Answer from the drawing. Dimensions are ordinates in mm from the lowest x, y and z of the part. A direction names the side the tool comes from. Give positions to 0.01 mm unless a question says otherwise; leave off trailing zeros. Order: outer loops, then holes, each group sorted by start corner. A loop starts at its lowest first (then second) coordinate and runs counter-clockwise, first axis right, second up. Notation, with made-up numbers: M 18,76.25 L 32,76.25 A4 cw 32,80.25 Z; hole C 69.25,20.5 d4. An arc over 180 degrees is marked long. One line per item, written item: value.
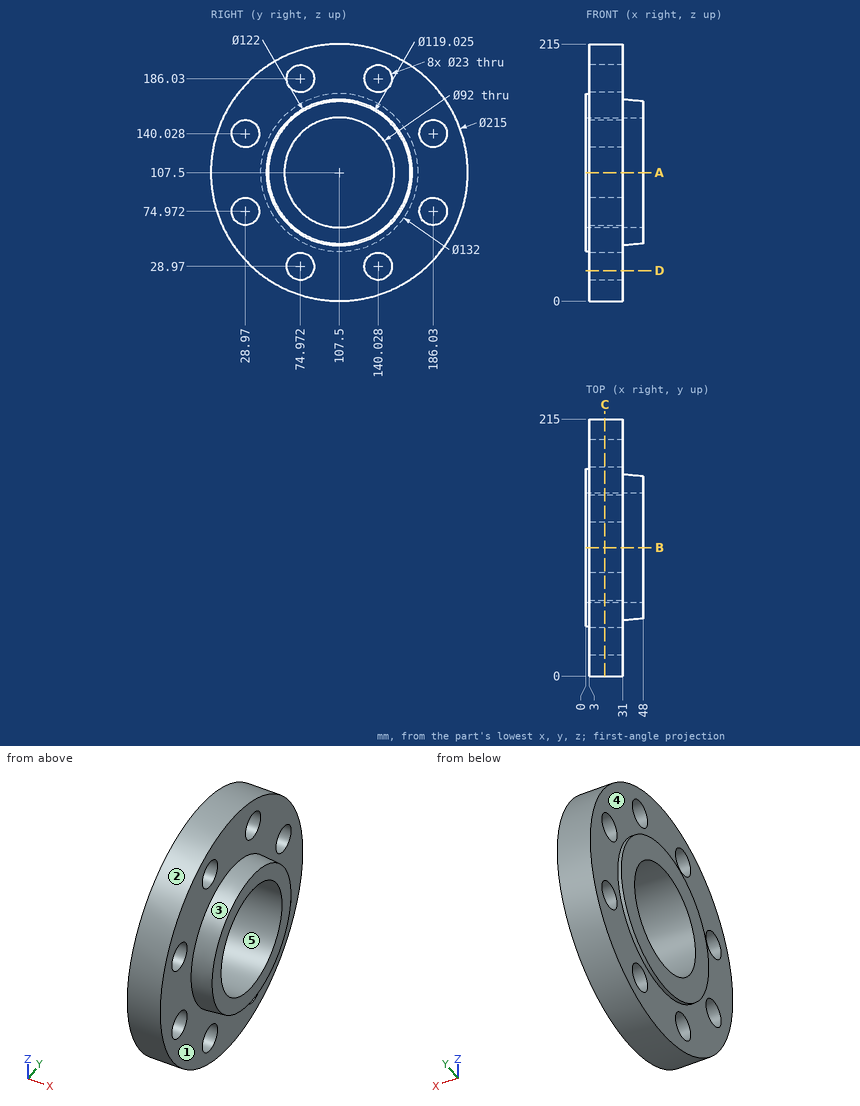
(1) Section C-C, the plane x = 16 is taken. Give the number of separate pieces and of enclosed holes in the cut face, then the cut area to 3 significant figures.
Findings:
separate pieces: 1
enclosed holes: 9
area: 26,300 mm^2
(2) Which of the six approach directions +Z, -Z, +X, -X, +Y, -Y give full straight-line access (tool end or side, diameter ignored) to the marked faces 1 and 2?
Findings:
face 1: +X
face 2: +X, -X
(3) Section A-A, the plane z = 107.5 is taken. Give the vertices of the cut face in (x, y).
Findings:
outline: M 0,41.5 L 3,41.5 L 3,0 L 31,0 L 31,46.5 L 48,47.99 L 48,61.5 L 0,61.5 Z; M 0,153.5 L 48,153.5 L 48,167.01 L 31,168.5 L 31,215 L 3,215 L 3,173.5 L 0,173.5 Z
(4) Determine the mould class of the marked faces 3, 4 and 5 for opening direction Z: pulls with the +Z half, pulls with the -Z half, needs draft (parallel to the pull), parting line crosses it, or undercut.
Findings:
face 3: parting line crosses it
face 4: needs draft
face 5: undercut
(5) Given P1, Ø3, axis at y = 51.5, z = 187, coming from the -X side; P2, Ø1, axis at x = 33.5, y = 53.5, coming from the +Z side; P3, Ø12, axis at x = 28.5, z = 175.5, coming from the -Y side; P4, Ø18.5, axis at y = 186.03, z = 140.03, coming from the -X side, each flat-ended and moving along its own axis, determine where each tip first touches the part or whether it passes through.
Findings:
P1: stops at x = 3
P2: stops at z = 136.35
P3: stops at y = 19.68
P4: passes through
(6) Find the intervals of material crossed by probe 1 along Y at (x, z) = (17.5, 27) (1 decimal); probe 2 along Y at (x, z) = (21, 34) (1 decimal); probe 3 along Z at (x, y) = (21, 68.5) (1 decimal), in increasing order. Write a range as from..to.
Findings:
probe 1: y = 36.3..63.6, 86.3..128.7, 151.4..178.7
probe 2: y = 29.1..64.6, 85.3..129.7, 150.4..185.9
probe 3: z = 7.3..19.5, 38.5..83.1, 131.9..176.5, 195.5..207.7
(7) Section D-D, the plane z = 25.5 is taken. Give the vertices of the cut face in (x, y) (1 decimal), then the cut area to 4 significant figures.
Findings:
outline: M 3,38 L 31,38 L 31,64 L 3,64 Z; M 3,85.9 L 31,85.9 L 31,129.1 L 3,129.1 Z; M 3,151 L 31,151 L 31,177 L 3,177 Z
area: 2,665 mm^2
